CAD build for the part. Positions are in the model's coordinates, mm. A direction names the side the tool comes from. Coordinates: 2 decimals unless noted, no trailing zeros. Loops run counter-clockwise (first coordinate to the right, second up) from the corner with the lowest first, then second, coordinate; pieces in that order, holes last.
1) Saw through at D-D, the plane x = -7. Write the cut outline in (y, z), and give its area (3 significant figures).
2) Saw through at B-B, the plane z = -123. Write the cut outline in (x, y), and give its area (3 significant figures).
3) Two-plate mould, pull along Z, no slides. Class faces 4 (the flat face through (52, 150, -10.946)), 5 (the cylindrical face through (-56.245, 10.14, -102.596)), 6 (the flat face through (-1, 84, 75)), 7 (the flat face through (0, 150, -51)): +Z half, -Z half, draft (parallel to the pull), parting line (faces both ways), or undercut.
4) Wall check: line 1 along Z through (x, y) = (14.5, 154.5); line 2 along Z through (x, y) = (-86, 106.5); line 3 along Y through (x, z) = (30.5, -140). Give the ranges that are in metal, low to high.
5) Which spindle directions (+Z, -Z, +X, -X, +Y, -Y) get a long thin tool onto all of the face, cutting with end or side? Do faces 1 (the flat face through (-43, 130, 1)), 2 (the flat face through (1, 20, -114)), 3 (the flat face through (-56, 110, -60)). Say none if no direction does.
6) Pin check, flat tips, straight feed: pin 1 Ø12 at (x, y) = (64.5, 40) entering from -Z; pin 2 Ø23.5 at (x, z) = (12, -123) entering from +Y; pin 3 Ø23.5 at (x, z) = (-55.79, -60) entering from +Y; pin 4 Ø20 at (x, z) = (-60, -114.52) entering from +Y. Stop position of each tip, or through.
7) Saw through at C-C, the plane z = -44.5. Write the cut outline in (x, y), and give its area (3 significant figures).
8) Saw through at A-A, the plane x = 60. Write the cut outline in (y, z).
```python
from build123d import *

# Parameters (mm, degrees)
SKETCH_1_W               = 200
SKETCH_1_H               = 150
EXTRUDE_1_DEPTH          = 180
CUT_EXTRUDE_1_DEPTH      = 100
SKETCH_3_W               = 120
SKETCH_3_H               = 16.18209701
CUT_EXTRUDE_2_DEPTH      = 50
SKETCH_4_R               = 9
CUT_EXTRUDE_3_DEPTH      = 20
SKETCH_5_W               = 79.036616744
SKETCH_5_H               = 20
EXTRUDE_2_DEPTH          = 200
SKETCH_6_R               = 12.5
CUT_EXTRUDE_4_DEPTH      = 210
CUT_EXTRUDE_5_DEPTH      = 308.989889135
CUT_EXTRUDE_5_DEPTH_BACK = 308.989889135


with BuildPart() as part:
    # 草图1 → 凸台-拉伸1 (new body)
    with BuildSketch(Plane(origin=(0, 0, 0), x_dir=(1, 0, 0), z_dir=(0, 1, 0))):
        Rectangle(SKETCH_1_W, SKETCH_1_H)
    extrude(amount=EXTRUDE_1_DEPTH)

    # 草图2 → 切除-拉伸1 (cut, symmetric)
    with BuildSketch(Plane.XY):
        Polygon((-100, 180), (30, 180), (-20, 130), (-100, 130), align=None)
    extrude(amount=CUT_EXTRUDE_1_DEPTH, both=True, mode=Mode.SUBTRACT)

    # 草图3 → 切除-拉伸2 (cut)
    with BuildSketch(Plane(origin=(0, 180, 0), x_dir=(1, 0, 0), z_dir=(0, 1, 0))):
        with Locations((40, 19.036616744)):
            Rectangle(SKETCH_3_W, SKETCH_3_H)
    extrude(amount=-CUT_EXTRUDE_2_DEPTH, mode=Mode.SUBTRACT)

    # 草图4 → 切除-拉伸3 (cut)
    with BuildSketch(Plane(origin=(0, 130, 0), x_dir=(1, 0, 0), z_dir=(0, 1, 0))):
        with Locations(Location((-55.786910577, 60, 0), (0, 0, 180))):
            Circle(SKETCH_4_R)
        with Locations(Location((-55.786910577, -60, 0), (0, 0, 180))):
            Circle(SKETCH_4_R)
    extrude(amount=-CUT_EXTRUDE_3_DEPTH, mode=Mode.SUBTRACT)

    # 草图5 → 凸台-拉伸2 (add)
    with BuildSketch(Plane(origin=(100, 0, 0), x_dir=(0, 0, -1), z_dir=(1, 0, 0))):
        with Locations((114.518308372, 10)):
            Rectangle(SKETCH_5_W, SKETCH_5_H)
    extrude(amount=-EXTRUDE_2_DEPTH)

    # 草图6 → 切除-拉伸4 (cut)
    with BuildSketch(Plane(origin=(0, 20, 0), x_dir=(1, 0, 0), z_dir=(0, 1, 0))):
        with Locations(Location((-60, 114.518308372, 0), (0, 0, 270))):
            Circle(SKETCH_6_R)
        with Locations(Location((60, 114.518308372, 0), (0, 0, 270))):
            Circle(SKETCH_6_R)
    extrude(amount=-CUT_EXTRUDE_4_DEPTH, mode=Mode.SUBTRACT)

    # 草图7 → 切除-拉伸5 (cut, two sides: drawn at the far end of the back side and taken through both)
    with BuildSketch(Plane.XY.offset(75).offset(-CUT_EXTRUDE_5_DEPTH_BACK)):
        Polygon((20, 170), (112.388945941, 170), (112.388945941, 195.821739968), (6.51381217, 195.821739968), align=None)
    extrude(amount=CUT_EXTRUDE_5_DEPTH + CUT_EXTRUDE_5_DEPTH_BACK, mode=Mode.SUBTRACT)


solid = part.part
```
Data:
1. outline: (0, -154.04) - (20, -154.04) - (20, -75) - (143, -75) - (143, -27.13) - (130, -27.13) - (130, -10.95) - (143, -10.95) - (143, 75) - (0, 75) - close
1. area: 22,800 mm2
2. outline: (-100, 0) - (-69.18, 0) - (-69.18, 20) - (-100, 20) - close; (-50.82, 0) - (50.82, 0) - (50.82, 20) - (-50.82, 20) - close; (69.18, 0) - (100, 0) - (100, 20) - (69.18, 20) - close
2. area: 3,270 mm2
3. face 4: undercut
3. face 5: undercut
3. face 6: +Z half
3. face 7: draft
4. line 1: z = -75 to -27.13, -10.95 to 75
4. line 2: z = -75 to 75
4. line 3: y = 0 to 20
5. face 1: -X, +Y
5. face 2: -Z, +X, -X, +Y
5. face 3: +Y
6. pin 1: stops at z = -75
6. pin 2: stops at y = 20
6. pin 3: stops at y = 130
6. pin 4: passes through
7. outline: (-100, 0) - (100, 0) - (100, 170) - (20, 170) - (-20, 130) - (-100, 130) - close
7. area: 30,000 mm2
8. outline: (0, -154.04) - (20, -154.04) - (20, -127.02) - (0, -127.02) - close; (0, -102.02) - (20, -102.02) - (20, -75) - (170, -75) - (170, -27.13) - (130, -27.13) - (130, -10.95) - (170, -10.95) - (170, 75) - (0, 75) - close
